```python
from build123d import *

# Parameters (mm, degrees)
SKETCH1_W                      = 8.5
SKETCH1_H                      = 113.5
BOSS_EXTRUDE1_DEPTH            = 8.5
SKETCH12_W                     = 8.5
SKETCH12_H                     = 3
BOSS_EXTRUDE2_DEPTH            = 15
M2X0_4_TAPPED_HOLE1_D          = 1.6
M2X0_4_TAPPED_HOLE1_DEPTH      = 5.2
M2X0_4_TAPPED_HOLE1_TIP        = 0.480688495
F_2_2_2_2_DIAMETER_HOLE1_D     = 2.2
F_2_2_2_2_DIAMETER_HOLE1_DEPTH = 13
SKETCH25_W                     = 8.5
SKETCH25_H                     = 3
BOSS_EXTRUDE3_DEPTH            = 10
SKETCH30_W                     = 5.5
SKETCH30_H                     = 8.5
CUT_EXTRUDE2_DEPTH             = 5
SKETCH31_R                     = 1
CUT_EXTRUDE3_DEPTH             = 2
FILLET1_R                      = 1
M2X0_4_TAPPED_HOLE3_D          = 1.6
M2X0_4_TAPPED_HOLE3_DEPTH      = 3
M2X0_4_TAPPED_HOLE2_D          = 2
M2X0_4_TAPPED_HOLE2_DEPTH      = 5.2
M2X0_4_TAPPED_HOLE2_TIP        = 0.600860619
SKETCH45_W                     = 1.6
SKETCH45_H                     = 10
SKETCH45_W_2                   = 15
SKETCH45_H_2                   = 1.6
CUT_EXTRUDE4_DEPTH             = 10


with BuildPart() as part:
    # Sketch1 → Boss-Extrude1 (new body)
    with BuildSketch(Plane.XY):
        with Locations((4.25, -56.75)):
            Rectangle(SKETCH1_W, SKETCH1_H)
    extrude(amount=BOSS_EXTRUDE1_DEPTH)

    # Sketch12 → Boss-Extrude2 (add)
    with BuildSketch(Plane(origin=(8.5, 0, 0), x_dir=(0, 0, -1), z_dir=(1, 0, 0))):
        with Locations((-4.25, -100.5)):
            Rectangle(SKETCH12_W, SKETCH12_H)
    extrude(amount=BOSS_EXTRUDE2_DEPTH)

    # M2x0.4 Tapped Hole1
    with Locations(Plane(origin=(0, -99, 0), x_dir=(1, 0, 0), z_dir=(0, 1, 0))):
        with Locations((19.5, -2.75)):
            Hole(M2X0_4_TAPPED_HOLE1_D / 2, depth=M2X0_4_TAPPED_HOLE1_DEPTH)
            with Locations((0, 0, -(M2X0_4_TAPPED_HOLE1_DEPTH + M2X0_4_TAPPED_HOLE1_TIP / 2))):  # 118° drill point
                Cone(0, M2X0_4_TAPPED_HOLE1_D / 2, M2X0_4_TAPPED_HOLE1_TIP, mode=Mode.SUBTRACT)

    # Ø2.2 (2.2) Diameter Hole1
    with Locations(Plane(origin=(0, -99, 0), x_dir=(1, 0, 0), z_dir=(0, 1, 0))):
        with Locations((15.5, -4.2)):
            Hole(F_2_2_2_2_DIAMETER_HOLE1_D / 2, depth=F_2_2_2_2_DIAMETER_HOLE1_DEPTH)

    # Sketch19 → CBORE for M2 Socket Head Cap Screw1 (revolve, cut)
    with BuildSketch(Plane(origin=(0, -9.5, 4.25), x_dir=(0, 0, 1), z_dir=(0, 1, 0))):
        Polygon((0, 0), (0, 23.500025), (1.2, 23.500025), (1.2, 2.025), (1.225, 2), (2.2, 2), (2.2, 0), align=None)
    revolve(axis=Axis((-6.35, -9.5, 4.25), (1, 0, 0)), mode=Mode.SUBTRACT)

    # Sketch25 → Boss-Extrude3 (add)
    with BuildSketch(Plane(origin=(0, 0, 0), x_dir=(-1, 0, 0), z_dir=(0, 0, -1))):
        with Locations((-4.25, -100.5)):
            Rectangle(SKETCH25_W, SKETCH25_H)
    extrude(amount=BOSS_EXTRUDE3_DEPTH)

    # Sketch30 → Cut-Extrude2 (cut)
    with BuildSketch(Plane(origin=(0, 0, 0), x_dir=(-1, 0, 0), z_dir=(0, 0, -1))):
        with Locations((-4.25, -107.75)):
            Rectangle(SKETCH30_W, SKETCH30_H)
    extrude(amount=-CUT_EXTRUDE2_DEPTH, mode=Mode.SUBTRACT)

    # Sketch31 → Cut-Extrude3 (cut)
    with BuildSketch(Plane(origin=(0, -113.5, 0), x_dir=(-1, 0, 0), z_dir=(0, -1, 0))):
        with Locations((-4.25, -4.25)):
            Circle(SKETCH31_R)
    extrude(amount=-CUT_EXTRUDE3_DEPTH, mode=Mode.SUBTRACT)

    # Fillet1
    fillet1_edges = [part.edges().sort_by_distance(p)[0] for p in [
        (4.25, 0, 8.5),
        (0, -56.75, 8.5),
        (4.25, 0, 0),
        (4.25, -113.5, 0),
        (4.25, -113.5, 8.5),
        (0, 0, 4.25),
        (8.5, 0, 4.25),
        (8.5, -113.5, 4.25),
        (0, -113.5, 4.25),
        (5.25, -113.5, 4.25),
    ]]
    fillet(fillet1_edges, radius=FILLET1_R)

    # M2x0.4 Tapped Hole3
    with Locations(Plane(origin=(0, -99, 0), x_dir=(1, 0, 0), z_dir=(0, 1, 0))):
        with Locations((5.05, 5)):
            Hole(M2X0_4_TAPPED_HOLE3_D / 2, depth=M2X0_4_TAPPED_HOLE3_DEPTH)

    # M2x0.4 Tapped Hole2
    with Locations(Plane(origin=(0, 0, 0), x_dir=(-1, 0, 0), z_dir=(0, 0, -1))):
        with Locations((-5.05, -26.8), (-5.05, -84.2), (-5.05, -31.1), (-5.05, -79.9)):
            Hole(M2X0_4_TAPPED_HOLE2_D / 2, depth=M2X0_4_TAPPED_HOLE2_DEPTH)
            with Locations((0, 0, -(M2X0_4_TAPPED_HOLE2_DEPTH + M2X0_4_TAPPED_HOLE2_TIP / 2))):  # 118° drill point
                Cone(0, M2X0_4_TAPPED_HOLE2_D / 2, M2X0_4_TAPPED_HOLE2_TIP, mode=Mode.SUBTRACT)

    # Sketch43 → CBORE for M1.6 Socket Head Cap Screw1 (revolve, cut)
    with BuildSketch(Plane(origin=(4.25, -104.85, 8.5), x_dir=(0, -1, 0), z_dir=(1, 0, 0))):
        Polygon((0, 0), (0, 18.500025), (0.9, 18.500025), (0.9, 1.625), (0.925, 1.6), (1.75, 1.6), (1.75, 0), align=None)
    revolve(axis=Axis((4.25, -104.85, 14.85), (0, 0, -1)), mode=Mode.SUBTRACT)

    # Sketch45 → Cut-Extrude4 (cut)
    with BuildSketch(Plane(origin=(0, -99, 0), x_dir=(1, 0, 0), z_dir=(0, 1, 0))):
        with Locations((0.8, 5)):
            Rectangle(SKETCH45_W, SKETCH45_H)
        with Locations((16, -7.7)):
            Rectangle(SKETCH45_W_2, SKETCH45_H_2)
    extrude(amount=-CUT_EXTRUDE4_DEPTH, mode=Mode.SUBTRACT)


solid = part.part
```
Geometry check sheet. Reference: the model listing, model coordinates, mm. A direction names the side the tool comes from. Coordinates: 2 decimals unless noted, no trailing zeros. Write each loop counter-clockwise with the first axis right and the second up, starting at its lowest first coordinate (ties: lowest second). Pieces come first, ordered by that corner, then holes. Notation, with made-up numbers: M 58,-20.5 L 115,-20.5 A27 cw 115,-2.5 Z; hole C 42.25,-8.75 d8. An arc over 180 degrees is marked long. Use one line per item in the form item = value. Start each with the question number.
1) Thickness scan on probe 1 along Y at (x, z) = (5.05, 2.05); probe 2 along X at (y, z) = (-104.85, 5.4); probe 3 along Z at (x, y) = (19.5, -100.5). Record the ranges inside material, lowest first. Write a range as from..to.
2) Section check A-A on x = 15.5. Enter the section's corners in (y, z), and give its area (3 significant figures).
3) Section check B-B on y = -9.5. Enter the section's corners in (x, z) (3 decimals), and give its area (3 significant figures).
4) Go/stop test with flat-tipped pins: pin 1 Ø5.5 at (x, z) = (19.5, 3) entering from -Y; pin 2 Ø1.8 at (x, y) = (5.05, -26.8) entering from -Z; pin 3 Ø2.5 at (x, y) = (3, -50.5) entering from -Z. Record where each tip stops, or that it passes through.
5) Section check C-C on y = -66.5. Enter the section's corners in (x, z), and give its area (3 significant figures).
6) Release check for a two-part mould opening along X. For faces 5 (the flat face through (2, -9.5, 2.8)), 6 (the cylindrical face through (3.98, -105.71, 5.95)), 7 (the flat face through (16, -102, 3)) record: pulls with the +X half, pulls with the -X half, needs draft (parallel to the pull), parting line crosses it, or undercut.
7) Set-up check for faces 1 (the cylindrical face through (4.2, -103.1, 7.7)), 2 (the flat face through (4, -112, 2)), 3 (the flat face through (1.6, -100, -5)), 4 (the cylindrical face through (0.99, -10.16, 6.35)): record each of +Z, -Z, +X, -X, +Y, -Y from which the full face is reachable in a straight line by a thin tool's end or side.
8) Section check D-D on z = -7. Enter the section's corners in (x, y), and give its area (3 significant figures).
Responses:
q1.probe_1 = -113.5..-112, -103.5..-85.2, -83.2..-80.9, -78.9..-32.1, -30.1..-27.8, -25.8..0
q1.probe_2 = 0..3.35, 5.15..8.5
q1.probe_3 = 0..1.95, 3.55..6.9
q2.outline = M -102,0 L -99,0 L -99,3.1 L -102,3.1 Z; M -102,5.3 L -99,5.3 L -99,6.9 L -102,6.9 Z
q2.area = 14.1 mm2
q3.outline = M 0,0 L 8.5,0 L 8.5,3.05 L 2.025,3.05 L 2,3.025 L 2,2.05 L 0,2.05 Z; M 0,6.45 L 2,6.45 L 2,5.475 L 2.025,5.45 L 8.5,5.45 L 8.5,8.5 L 1,8.5 A1 ccw 0,7.5 Z
q3.area = 47.6 mm2
q4.pin_1 = -102
q4.pin_2 = 5.26
q4.pin_3 = 0
q5.outline = M 0,0 L 8.5,0 L 8.5,8.5 L 1,8.5 A1 ccw 0,7.5 Z
q5.area = 72.0 mm2
q6.face_5 = pulls with the -X half
q6.face_6 = undercut
q6.face_7 = needs draft
q7.face_1 = +Z
q7.face_2 = -Z
q7.face_3 = -Z, -X, +Y, -Y
q7.face_4 = -X
q8.outline = M 1.6,-102 L 8.5,-102 L 8.5,-99 L 1.6,-99 Z
q8.area = 20.7 mm2
